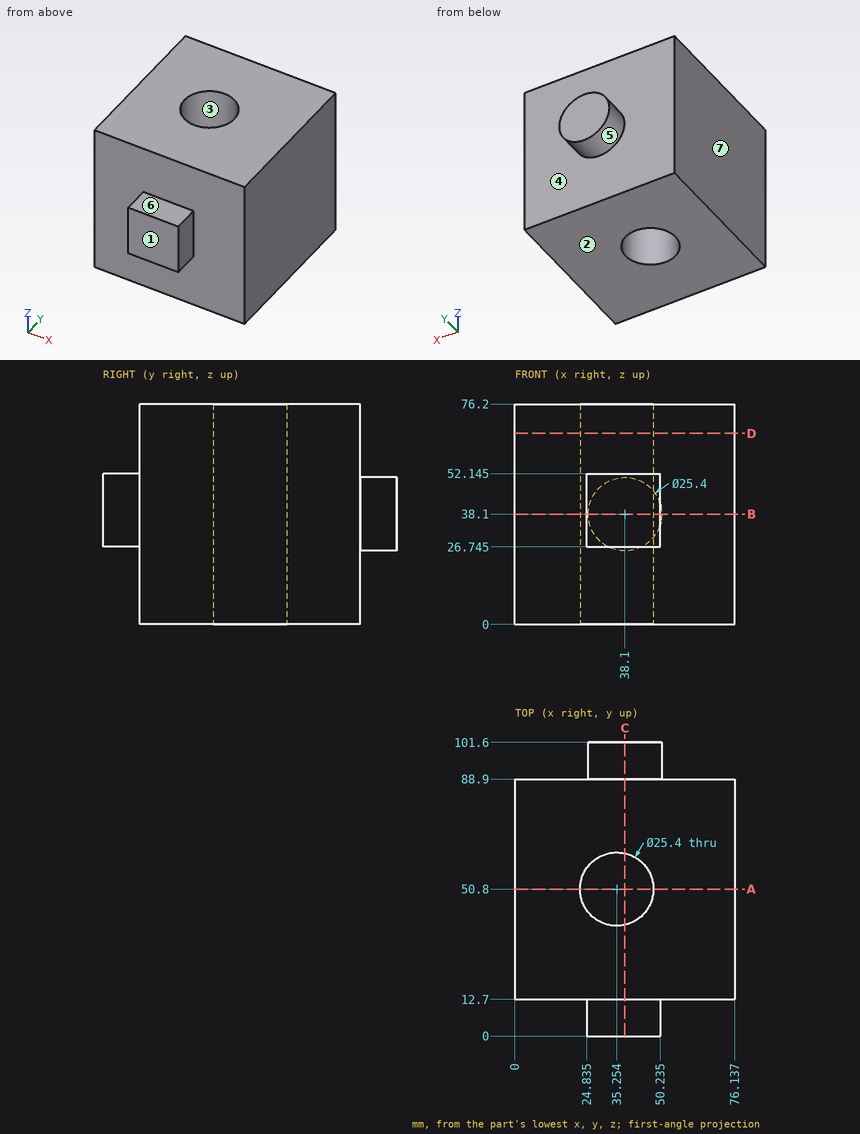
Geometry check sheet. Reference: drawing and pictorial views, mm from the part's lowest x, y, z. A direction names the side the tool comes from. Give positions to 0.01 mm unless a question says otherwise; leave off trailing zeros. Write each loop counter-clockwise with the first axis right and the second up, starting at its lowest first coordinate (ties: lowest second). Pieces come first, ordered by that corner, then holes. Notation, with made-up numbers: (15, 70) -> (71, 70) arc R12 ccw to (71, 76) -> close; hole circle Ø5 at (72.5, 37.5). An arc over 180 degrees is marked (long way). One line per item, written item: value. Start each with the question number.
Item 1: Section check C-C on x = 38.1. Record the cut outline in (y, z) (1 decimal).
Item 2: Section check D-D on z = 66. Record the cut outline in (x, y), then the cut area to 4 significant figures.
Item 3: Section check A-A on y = 50.8. Record the cut outline in (x, z), then the cut area to 3 significant figures.
Item 4: Tool access check on the marked faces 5, 6 and 7. Record the directions out of +Z, -Z, +X, -X, +Y, -Y that give a thin tool (end or side, any length) a straight path to the whole face; none if there is none.
Item 5: Draft check along Y on the marked faces 1, 2, 3 and 4. Enter one of: +Y half, -Y half, draft (parallel to the pull), parting line (faces both ways), or undercut.
Item 6: Section check B-B on z = 38.1. Record the cut outline in (x, y) (1 decimal).
Item 7: Material ranges on probe 1 along X at (y, z) = (50, 22); probe 2 along Y at (x, z) = (49, 10); probe 3 along Y at (x, z) = (34.5, 72.5), recorded low to high. Write a range as from..to.
Item 8: Gauge pin test, flat ends, axial feed: pin 1 (1.5 mm diameter, centred on x = 63.5, z = 47, fed in from +Y); pin 2 (6.5 mm diameter, centred on x = 31, y = 7, fed in from -Z) (1 decimal); pin 3 (10 mm diameter, centred on y = 4, z = 37, fed in from +X) (1 decimal). Record the tip position at first contact, or that the pin passes through.
Results list:
1. outline: (0, 26.7) -> (12.7, 26.7) -> (12.7, 0) -> (38.4, 0) -> (38.4, 76.2) -> (12.7, 76.2) -> (12.7, 52.1) -> (0, 52.1) -> close; (63.2, 0) -> (88.9, 0) -> (88.9, 25.4) -> (101.6, 25.4) -> (101.6, 50.8) -> (88.9, 50.8) -> (88.9, 76.2) -> (63.2, 76.2) -> close
2. outline: (0, 12.7) -> (76.14, 12.7) -> (76.14, 88.9) -> (0, 88.9) -> close; hole circle Ø25.4 at (35.25, 50.8)
2. area: 5,295 mm²
3. outline: (0, 0) -> (22.55, 0) -> (22.55, 76.2) -> (0, 76.2) -> close; (47.95, 0) -> (76.14, 0) -> (76.14, 76.2) -> (47.95, 76.2) -> close
3. area: 3,870 mm²
4. face 5: +Y
4. face 6: +Z, +X, -X, -Y
4. face 7: +Z, -Z, -X, +Y, -Y
5. face 1: -Y half
5. face 2: draft
5. face 3: undercut
5. face 4: +Y half
6. outline: (0, 12.7) -> (24.8, 12.7) -> (24.8, 0) -> (50.2, 0) -> (50.2, 12.7) -> (76.1, 12.7) -> (76.1, 88.9) -> (50.8, 88.9) -> (50.8, 101.6) -> (25.4, 101.6) -> (25.4, 88.9) -> (0, 88.9) -> close; hole circle Ø25.4 at (35.3, 50.8)
7. probe 1: 0..22.58, 47.93..76.14
7. probe 2: 12.7..88.9
7. probe 3: 12.7..38.12, 63.48..88.9
8. pin 1: y = 88.9
8. pin 2: z = 26.7
8. pin 3: x = 50.2
